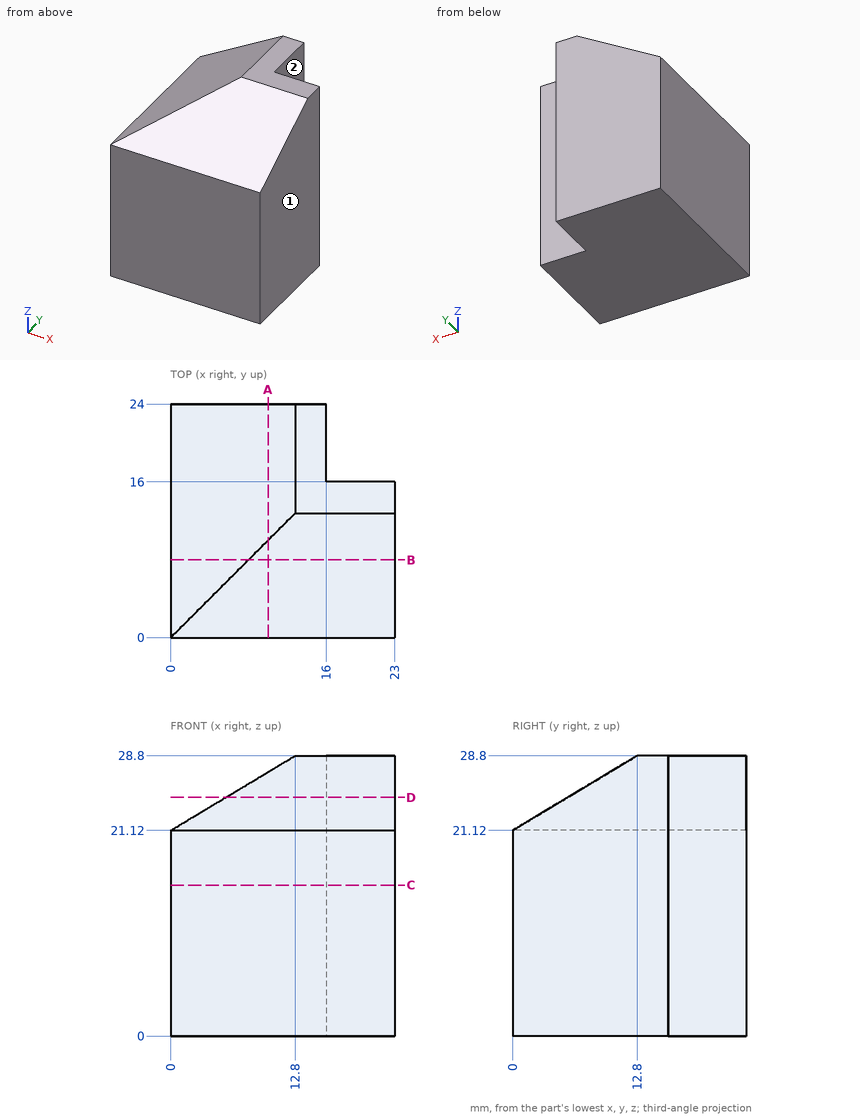
Print and shaded views of the part. All mm, measured from the part's lowest x, y and z. A direction names the side the tool comes from. Round coordinates to 2 decimals unless told otherwise and drop trailing zeros. Write each loop counter-clockwise with the first axis right and the second up, starting at its lowest first coordinate (ties: lowest second). Pieces come first, ordered by that corner, then holes. Notation, with made-up numbers: (21, 84) - (73, 84) arc R32 ccw to (73, 116) - close; hole circle Ø4 at (-23.5, -29). An arc over 180 degrees is marked (long way). One line per question, with ' | ' between items.
1. Band-saw the part on C-C, the plane z = 15.5. Write the cut outline in (x, y).
Results are:
outline: (0, 0) - (23, 0) - (23, 16) - (16, 16) - (16, 24) - (0, 24) - close
2. Drill centre lines: line 1 along X through (y, z) = (19, 14.75); line 2 along Z through (x, y) = (12.5, 2.5). Where is each one in solid material? Low to high. Write a range as from..to.
Results are:
line 1: 0..16 | line 2: 0..22.62
3. Band-saw the part on B-B, the plane y = 8. Write the cut outline in (x, z), and give its area (3 significant figures).
Results are:
outline: (0, 0) - (23, 0) - (23, 25.92) - (8, 25.92) - (0, 21.12) - close | area: 577 mm^2
4. Tool access for the marked faces 1 and 2: list every direction of +Z, -Z, +X, -X, +Y, -Y with a clear straight run to the whole face (end or side of a thin tool).
Results are:
face 1: +Z, -Z, +X, +Y, -Y | face 2: +Z, -Z, +X, +Y
5. Band-saw the part on D-D, the plane z = 24.5. Write the cut outline in (x, y).
Results are:
outline: (5.63, 5.63) - (23, 5.63) - (23, 16) - (16, 16) - (16, 24) - (5.63, 24) - close
6. Band-saw the part on A-A, the plane x = 10. Write the cut outline in (y, z).
Results are:
outline: (0, 0) - (24, 0) - (24, 27.12) - (10, 27.12) - (0, 21.12) - close
7. Drop flat-ended pins along their axis: pin 1 Ø4 at (y, z) = (21.5, 21.5) entering from +X; pin 2 Ø1 at (x, y) = (9.5, 19) entering from +Z; pin 3 Ø1 at (y, z) = (10, 24.5) entering from -X. Give the stop position or say it passes through.
Results are:
pin 1: x = 16 | pin 2: z = 27.12 | pin 3: x = 4.8
